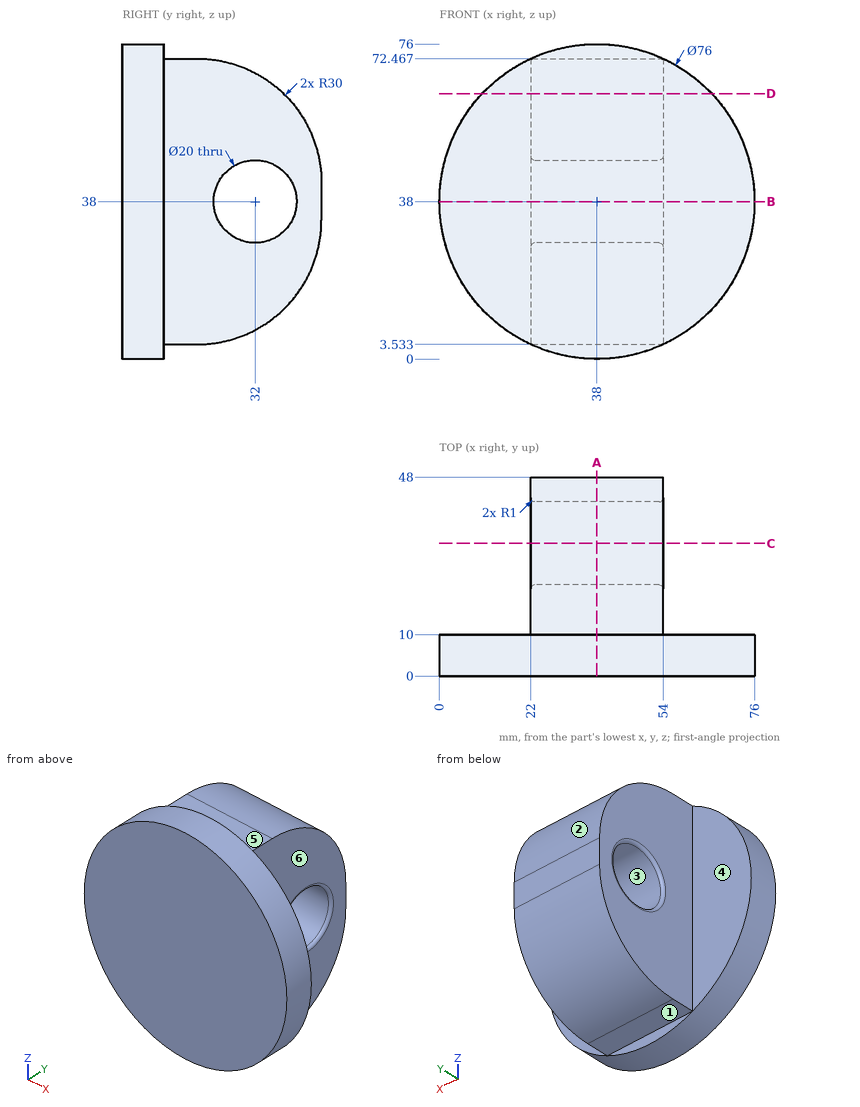
Geometry: see drawing. Coordinates: mm, zero at the bounding-box minimum. A direction names the side the tool comes from. Coordinates: 2 decimals unless noted, no trailing zeros. Loops run counter-clockwise (first coordinate to the right, second up) from the corner with the lowest first, then second, coordinate; pieces in that order, holes last. Notation, with made-up numbers: (33, 51.5) -> (56, 51.5) arc R37 ccw to (56, 88.5) -> close; hole circle Ø8 at (3.5, -16). An arc over 180 degrees is marked (long way). Use a Markdown table: item, result.
1) Cut plane D-D (z = 64). Return the cut outline in (x, y), then the cut area to 3 significant figures.
Results found:
| item | result |
|---|---|
| outline | (10.29, 0) -> (65.71, 0) -> (65.71, 10) -> (54, 10) -> (54, 38.89) -> (22, 38.89) -> (22, 10) -> (10.29, 10) -> close |
| area | 1,480 mm2 |
2) Cut plane B-B (z = 38). Return the cut outline in (x, y), then the cut area to 4 significant figures.
Results found:
| item | result |
|---|---|
| outline | (0, 0) -> (76, 0) -> (76, 10) -> (54, 10) -> (54, 21) arc R1 ccw to (53, 22) -> (23, 22) arc R1 ccw to (22, 21) -> (22, 10) -> (0, 10) -> close; (22, 43) arc R1 ccw to (23, 42) -> (53, 42) arc R1 ccw to (54, 43) -> (54, 48) -> (22, 48) -> close |
| area | 1,335 mm2 |
3) Material intervals for line 1 along Y through (x, z) = (46, 38); line 2 along X through (y, z) = (14, 27); line 3 along Y through (x, z) = (6.5, 40), sorted ascending. Write a range as from..to.
Results found:
| item | result |
|---|---|
| line 1 | y = 0..22, 42..48 |
| line 2 | x = 22..54 |
| line 3 | y = 0..10 |
4) Cut plane C-C (y = 32). Return the cut outline in (x, z).
Results found:
| item | result |
|---|---|
| outline | (22, 7) -> (54, 7) -> (54, 27) arc R1 ccw to (53, 28) -> (23, 28) arc R1 ccw to (22, 27) -> close; (22, 49) arc R1 ccw to (23, 48) -> (53, 48) arc R1 ccw to (54, 49) -> (54, 69) -> (22, 69) -> close |
5) Contact query for flat-ended pins moving along their axis: pin 1 (1.8 mm diameter, centred on x = 40.5, z = 73.5, fed in from +Y); pin 2 (2 mm diameter, centred on x = 31.5, y = 16.5, fed in from +Z); pin 3 (11.5 mm diameter, centred on y = 33.5, z = 36, fed in from -X); pin 4 (12 mm diameter, centred on y = 42, z = 34.5, fed in from -X). Output: stop coordinate, or through.
Results found:
| item | result |
|---|---|
| pin 1 | stops at y = 10 |
| pin 2 | stops at z = 72.47 |
| pin 3 | passes through |
| pin 4 | stops at x = 22 |
6) Access query for the marked faces 4, 5 and 6. Directions: +Z, -Z, +X, -X, +Y, -Y. A direction counts if a zero-diameter tool reaches every point of the face in a straight line with its end or side. Return the directions, or none.
Results found:
| item | result |
|---|---|
| face 4 | +Z, -Z, -X, +Y |
| face 5 | +Z, +X, -X, +Y |
| face 6 | +Z, -Z, +X, +Y |
7) Pull-direction query (Y, two-part tool) for the marked faces 1, 2 and 3; classes: released by +Y, released by -Y, zero draft, split by the parting line, or undercut.
Results found:
| item | result |
|---|---|
| face 1 | zero draft |
| face 2 | released by +Y |
| face 3 | undercut |
8) Cut plane A-A (x = 38). Return the cut outline in (y, z), then the cut area to 3 significant figures.
Results found:
| item | result |
|---|---|
| outline | (0, 0) -> (10, 0) -> (10, 3.53) -> (18, 3.53) arc R30 ccw to (48, 33.53) -> (48, 42.47) arc R30 ccw to (18, 72.47) -> (10, 72.47) -> (10, 76) -> (0, 76) -> close; hole circle Ø20 at (32, 38) |
| area | 2,680 mm2 |
